Here's how the part is built. I have some questions about the finished solid (model axes, mm). A direction names the side the tool comes from. Coordinates: 2 decimals unless noted, no trailing zeros. Write each loop counter-clockwise with the first axis right and the second up, starting at its lowest first coordinate (ties: lowest second). Pieces come first, ordered by that corner, then holes. Notation, with made-up numbers: (-15, 45.5) -> (38, 45.5) arc R29 cw to (38, 67.5) -> close; hole circle Ø1 at (5.25, 11). An arc over 180 degrees is marked (long way). Put each result on its own line as item: value. Start each with the question number.
Item 1: For pin 1 (12.5 mm diameter, centred on x = 16.5, z = -78, fed in from +Y) (3 decimals); pin 2 (3 mm diameter, centred on x = 31.5, y = 46, fed in from -Z); pin 3 (2 mm diameter, centred on x = 67.5, y = 16.5, fed in from +Z), each with a flat end and sliding along its axis, tell me the tip position at first contact or that it passes through.
Item 2: I want a section at A-A, the plane y = 56.5. List the corners of the cut face in (x, z) for me (3 decimals), then the cut area to 3 significant figures.
Item 3: I want a section at B-B, the plane x = -88.9. List the corners of the cut face in (y, z) for me (3 decimals), then the cut area to 3 significant figures.
Item 4: I want a section at C-C, the plane z = -46.5. List the corners of the cut face in (x, y) for me (3 decimals), then the cut area to 3 significant figures.
Item 5: I want a section at D-D, the plane x = 51. List the corners of the cut face in (y, z) for me (3 decimals), then the cut area to 3 significant figures.
Item 6: I need wall thicknesses on line 1 (X direction, y = 29.5, z = 11) (3 decimals); line 2 (Z direction, x = -66, y = 42.5); line 3 (Z direction, x = 88, y = 3). Which ranges of each line are inside material? Lowest first, please. Write a range as [from, to].
Item 7: On a 3-axis mill with a long thin cutter (end or side, diameter ignored), from which of +Z, -Z, +X, -X, +Y, -Y can I reach the whole of each face in a straight line? I mean faces 1 (the face through (-1, 9.525, 74)), 2 (the face through (-1, 9.525, -1)), 3 (the face through (-1, 9.525, -75)). Say none if no direction works.
Item 8: If we mould it in two halves opening along X, with no side actions, what happens to faces 4 (the face through (85.416, 4.829, -75.45)), 5 (the face through (-1, 36, 61.976)), 6 (the face through (101.6, 32, 1))? For each: released by +X, released by -X, zero draft, split by the parting line, or undercut.
from build123d import *

# Parameters (mm, degrees)
SKETCH2_W              = 203.2
SKETCH2_H              = 123.952
MAIN_BLOCK_DEPTH       = 63.5
SHELL_T                = -9.525
SKETCH6_W              = 203.2
SKETCH6_H              = 25.4
SKETCH6_R              = 3.5687
MOUNTING_FLANGES_DEPTH = 9.525


with BuildPart() as part:
    # Sketch2 → Main Block (new body)
    with BuildSketch(Plane(origin=(0, 0, 0), x_dir=(1, 0, 0), z_dir=(0, 1, 0))):
        Rectangle(SKETCH2_W, SKETCH2_H)
    extrude(amount=MAIN_BLOCK_DEPTH)

    # Shell
    shell_openings = [part.faces().sort_by_distance(p)[0] for p in [
        (0, 63.5, 0),
    ]]
    offset(amount=SHELL_T, openings=shell_openings, kind=Kind.INTERSECTION)

    # Sketch6 → Mounting Flanges (add)
    # profile 1 of 2: a face of its own
    with BuildSketch(Plane(origin=(0, 9.525, 0), x_dir=(1, 0, 0), z_dir=(0, 1, 0))):
        with Locations((0, 74.676)):
            Rectangle(SKETCH6_W, SKETCH6_H)
        with Locations(Location((-88.9, 74.676, 0), (0, 0, 270))):
            Circle(SKETCH6_R, mode=Mode.SUBTRACT)
        with Locations(Location((88.9, 74.676, 0), (0, 0, 270))):
            Circle(SKETCH6_R, mode=Mode.SUBTRACT)
    # profile 2 of 2: a face of its own
    with BuildSketch(Plane(origin=(0, 9.525, 0), x_dir=(1, 0, 0), z_dir=(0, 1, 0))):
        with Locations((0, -74.676)):
            Rectangle(SKETCH6_W, SKETCH6_H)
        with Locations(Location((88.9, -74.676, 0), (0, 0, 270))):
            Circle(SKETCH6_R, mode=Mode.SUBTRACT)
        with Locations(Location((-88.9, -74.676, 0), (0, 0, 270))):
            Circle(SKETCH6_R, mode=Mode.SUBTRACT)
    extrude(amount=-MOUNTING_FLANGES_DEPTH)


solid = part.part
Calculated:
1. pin 1: stops at y = 9.525
1. pin 2: stops at z = -61.98
1. pin 3: stops at z = 61.98
2. outline: (-101.6, -61.976) -> (101.6, -61.976) -> (101.6, 61.976) -> (-101.6, 61.976) -> close; hole (-92.075, -52.451) -> (92.075, -52.451) -> (92.075, 52.451) -> (-92.075, 52.451) -> close
2. area: 5,870 mm2
3. outline: (0, -87.376) -> (9.525, -87.376) -> (9.525, -78.245) -> (0, -78.245) -> close; (0, -71.107) -> (9.525, -71.107) -> (9.525, -61.976) -> (63.5, -61.976) -> (63.5, -52.451) -> (9.525, -52.451) -> (9.525, 52.451) -> (63.5, 52.451) -> (63.5, 61.976) -> (9.525, 61.976) -> (9.525, 71.107) -> (0, 71.107) -> close; (0, 78.245) -> (9.525, 78.245) -> (9.525, 87.376) -> (0, 87.376) -> close
3. area: 2,560 mm2
4. outline: (-101.6, 0) -> (101.6, 0) -> (101.6, 63.5) -> (92.075, 63.5) -> (92.075, 9.525) -> (-92.075, 9.525) -> (-92.075, 63.5) -> (-101.6, 63.5) -> close
4. area: 2,960 mm2
5. outline: (0, -87.376) -> (9.525, -87.376) -> (9.525, -61.976) -> (63.5, -61.976) -> (63.5, -52.451) -> (9.525, -52.451) -> (9.525, 52.451) -> (63.5, 52.451) -> (63.5, 61.976) -> (9.525, 61.976) -> (9.525, 87.376) -> (0, 87.376) -> close
5. area: 2,690 mm2
6. line 1: x = [-101.6, -92.075], [92.075, 101.6]
6. line 2: z = [-61.98, -52.45], [52.45, 61.98]
6. line 3: z = [-87.38, -78.13], [-71.22, 71.22], [78.13, 87.38]
7. face 1: +Z, +X, -X, +Y
7. face 2: +Y
7. face 3: -Z, +X, -X, +Y
8. face 4: undercut
8. face 5: zero draft
8. face 6: released by +X
